Here's how the part is built. I have some questions about the finished solid (model axes, mm). Coordinates: 2 decimals unless noted, no trailing zeros. Loops run counter-clockwise (first coordinate to the right, second up) from the corner with the lowest first, then second, coordinate; pieces in that order, holes last. Notation, with made-up numbers: (2.5, 89.5) -> (9.5, 89.5) arc R25 cw to (9.5, 115.5) -> close; hole circle Ø4 at (80, 10). An arc over 180 degrees is marked (long way). Answer as a JSON object with one key per item and string values. Group by question number.
Q1. Thinking about a two-plate mould opening in Z: for faces 1 (the flat face through (4.08, -3.944, -39.063)), 2 (the cylindrical face through (31.66, -3.94, 40.48)), 3 (the cylindrical face through (29.915, -3.944, -27.252)), which applies, released by +Z, released by -Z, zero draft, split by the parting line, or undercut?
Q2. I want a section at B-B on z = -15. Write out the boundary of the cut face in (x, y), then the cut area to 3 significant figures.
Q3. I need wall thicknesses on line 1 (Z direction, x = -26.5, y = -5.75); line 2 (X direction, y = -1, z = -26.5). Which ranges of each line are inside material? Lowest first, please.
Q4. I'm going to push flat-ended pins straight in: pin 1 (1 mm diameter, centred on y = -5, z = 29.5, fed in from -X); pin 2 (2 mm diameter, centred on x = 7, y = -4, fed in from +Z). Where does each tip first touch, or does it pass through?
Q5. I want a section at A-A on y = -4.25. Write out the boundary of the cut face in (x, z).
Q6. I want a section at C-C on x = 0. Write out the boundary of the cut face in (y, z).
Q7. I want a section at D-D on z = 28. Write out the boundary of the cut face in (x, y), then the cut area to 3 significant figures.
```python
from build123d import *

# Parameters (mm, degrees)
F0_R     = 4.5
F0_R_2   = 32.5
F1_DEPTH = 8


with BuildPart() as f1:
    # F0 (on Front) → F1 (new body)
    with BuildSketch(Plane.XZ):
        with BuildLine():
            Line((24.51391, 43.48609), (-33.48609, 34.51391))
            ThreePointArc((-33.48609, 34.51391), (-40.557157, 31.584978), (-43.48609, 24.51391))
            Line((-43.48609, 24.51391), (-34.51391, -33.48609))
            ThreePointArc((-34.51391, -33.48609), (-31.584978, -40.557157), (-24.51391, -43.48609))
            Line((-24.51391, -43.48609), (33.48609, -34.51391))
            ThreePointArc((33.48609, -34.51391), (40.557157, -31.584978), (43.48609, -24.51391))
            Line((43.48609, -24.51391), (34.51391, 33.48609))
            ThreePointArc((34.51391, 33.48609), (31.584978, 40.557157), (24.51391, 43.48609))
        make_face()
        with Locations((-24.51391, -33.48609)):
            Circle(F0_R, mode=Mode.SUBTRACT)
        with Locations((33.48609, -24.51391)):
            Circle(F0_R, mode=Mode.SUBTRACT)
        Circle(F0_R_2, mode=Mode.SUBTRACT)
        with Locations((-33.48609, 24.51391)):
            Circle(F0_R, mode=Mode.SUBTRACT)
        with Locations((24.51391, 33.48609)):
            Circle(F0_R, mode=Mode.SUBTRACT)
    extrude(amount=F1_DEPTH)


solid = f1.part
```
Result set:
{
 "1": {"face 1": "released by -Z", "face 2": "released by +Z", "face 3": "undercut"},
 "2": {"outline": "(-37.37, -8) -> (-28.83, -8) -> (-28.83, 0) -> (-37.37, 0) -> close; (28.83, -8) -> (42.01, -8) -> (42.01, 0) -> (28.83, 0) -> close", "area": "174 mm²"},
 "3": {"line 1": "z = -43.29 to -37.52, -29.45 to -18.81, 18.81 to 35.59", "line 2": "x = -35.59 to -18.81, 18.81 to 29.45, 37.52 to 43.29"},
 "4": {"pin 1": "stops at x = -42.42", "pin 2": "stops at z = 40.93"},
 "5": {"outline": "(-43.49, 24.51) -> (-34.51, -33.49) arc R10 ccw to (-24.51, -43.49) -> (33.49, -34.51) arc R10 ccw to (43.49, -24.51) -> (34.51, 33.49) arc R10 ccw to (24.51, 43.49) -> (-33.49, 34.51) arc R10 ccw to start; hole circle Ø9 at (-33.49, 24.51); hole circle Ø65 at (0, 0); hole circle Ø9 at (-24.51, -33.49); hole circle Ø9 at (24.51, 33.49); hole circle Ø9 at (33.49, -24.51)"},
 "6": {"outline": "(-8, -39.69) -> (0, -39.69) -> (0, -32.5) -> (-8, -32.5) -> close; (-8, 32.5) -> (0, 32.5) -> (0, 39.69) -> (-8, 39.69) -> close"},
 "7": {"outline": "(-42.86, -8) -> (-36.33, -8) -> (-36.33, 0) -> (-42.86, 0) -> close; (-30.64, -8) -> (-16.5, -8) -> (-16.5, 0) -> (-30.64, 0) -> close; (16.5, -8) -> (35.36, -8) -> (35.36, 0) -> (16.5, 0) -> close", "area": "316 mm²"}
}
